CAD build for the part. Positions are in the model's coordinates, mm. A direction names the side the tool comes from. Round coordinates to 2 decimals unless told otherwise and drop trailing zeros. Write each loop counter-clockwise with the first axis right and the second up, starting at its lowest first coordinate (ties: lowest second). Pieces come first, ordered by that corner, then holes. Notation, with made-up numbers: (-26.75, 74.5) -> (18.25, 74.5) arc R32 ccw to (18.25, 109.5) -> close; hole circle Ø8 at (-2, 84.5). An arc over 180 degrees is marked (long way). Put each result on its own line as item: value. Start each with the question number.
1. Saw through at C-C on x = 0.55. State how many separate pieces and enclosed holes the cut face has, and give its area (3 significant figures).
2. 3-axis set-ups, long thin cutter, end or side, ignore diameter. For faces 4 (the cylindrical face through (1.578, 148.765, -37.068)), 5 (the cylindrical face through (1.578, 84.895, -22.369)): which of +Z, -Z, +X, -X, +Y, -Y reach the whole face in a straight line?
3. Flat gauge pins, fed straight in: P1, Ø9.5, axis at y = 0, z = 0, coming from the +X side; P2, Ø1.5, axis at x = 1, y = 88, coming from the -Z side; P3, Ø1.6, axis at x = 2, y = 45.5, coming from the -Z side. Where does each tip first touch, or does it go through?
4. Drill centre lines: line 1 (Z direction, x = 2.55, y = 0); line 2 (Y direction, x = 2.15, z = -94.5); line 3 (Y direction, x = 2.85, z = -65.5). Where is each one in solid material? Low to high. Write a range as from..to.
5. Saw through at A-A on z = 0. List the corners of the cut face in (x, y), and give its area (3 significant figures).
6. Saw through at D-D on y = 83.5. List the corners of the cut face in (x, z).
7. Saw through at B-B on z = -97. List the corners of the cut face in (x, y).
8. Pull direction Z, two halves, no side cores. Call faces 1 (the cylindrical face through (2, 0, 6)), 2 (the flat face through (0, 114, -32)), 3 (the flat face through (1.578, -0.207, -15.487)): pulls with the +Z half, pulls with the -Z half, needs draft (parallel to the pull), parting line crosses it, or undercut.
from build123d import *

# Parameters (mm, degrees)
EXTRUDE1_DEPTH            = 3.2
SKETCH5_R                 = 6
CHASSIS_MOUNT_HOLES_DEPTH = 244.405812041
SKETCH6_R                 = 4
ENGINE_MOUNT_HOLES_DEPTH  = 244.405812041
SKETCH7_R                 = 6.5
SKETCH7_R_2               = 7.5
BOSS_CLEARANCE_DEPTH      = 244.405812041
FILLET1_R                 = 3
FILLET2_R                 = 2
FILLET4_R                 = 4


with BuildPart() as part:
    # Sketch4 → Extrude1 (new body)
    with BuildSketch(Plane(origin=(0, 0, 0), x_dir=(0, 0, -1), z_dir=(1, 0, 0))):
        with BuildLine():
            Line((57.561676807, 155.782132528), (157.015436102, 171.930964589))
            ThreePointArc((157.015436102, 171.930964589), (170.191569786, 165.878071941), (169.567790519, 151.39156416))
            ThreePointArc((169.567790519, 151.39156416), (167.864843482, 149.829218431), (165.697709708, 149.026420829))
            Line((165.697709708, 149.026420829), (86.516546247, 136.169357202))
            ThreePointArc((86.516546247, 136.169357202), (83.134642067, 136.199619503), (79.956239663, 137.355452467))
            ThreePointArc((79.956239663, 137.355452467), (57.745458436, 139.047132616), (42.376364081, 122.923500175))
            ThreePointArc((42.376364081, 122.923500175), (41.240179336, 120.412740542), (39.600266647, 118.197900576))
            ThreePointArc((39.600266647, 118.197900576), (25.651951648, 95.833503084), (20.780663371, 69.92998369))
            Line((20.780663371, 69.92998369), (20.780663371, 30.61290747))
            ThreePointArc((20.780663371, 30.61290747), (26.962955948, 18.753205297), (20.37053182, 7.116486634))
            Line((20.37053182, 7.116486634), (10.815904153, -7.21222708))
            ThreePointArc((10.815904153, -7.21222708), (-4.092243171, -12.339106447), (-12.982184032, 0.680367435))
            Line((-12.982184032, 0.680367435), (-11.728287792, 24.606132992))
            ThreePointArc((-11.728287792, 24.606132992), (-11.013879957, 26.397161442), (-9.356926136, 27.383399496))
            ThreePointArc((-9.356926136, 27.383399496), (4.476016858, 43.584120766), (-7.587711328, 61.142029063))
            ThreePointArc((-7.587711328, 61.142029063), (-9.132498235, 62.296063238), (-9.655779017, 64.1519562))
            ThreePointArc((-9.655779017, 64.1519562), (-0.849075896, 102.602883239), (20.462203873, 135.797177398))
            ThreePointArc((20.462203873, 135.797177398), (37.331902598, 148.908426775), (57.561676807, 155.782132528))
        make_face()
    extrude(amount=EXTRUDE1_DEPTH)

    # Sketch5 → chassis mount holes (cut, through all)
    with BuildSketch(Plane(origin=(0, 0, 0), x_dir=(0, 0, -1), z_dir=(1, 0, 0))):
        Circle(SKETCH5_R)
        with Locations((159.099025767, 159.099025767)):
            Circle(SKETCH5_R)
        with Locations((30.03123526, 126.997538987)):
            Circle(SKETCH5_R)
    extrude(amount=CHASSIS_MOUNT_HOLES_DEPTH, mode=Mode.SUBTRACT)

    # Sketch6 → engine mount holes (cut, through all)
    with BuildSketch(Plane(origin=(0, 0, 0), x_dir=(0, 0, -1), z_dir=(1, 0, 0))):
        with Locations((12.965088215, 18.997538987)):
            Circle(SKETCH6_R)
        with Locations((95.975539476, 147.520941453)):
            Circle(SKETCH6_R)
    extrude(amount=ENGINE_MOUNT_HOLES_DEPTH, mode=Mode.SUBTRACT)

    # Sketch7 → boss clearance (cut, through all)
    with BuildSketch(Plane(origin=(0, 0, 0), x_dir=(0, 0, -1), z_dir=(1, 0, 0))):
        with Locations((139.146474391, 144.715156547)):
            Circle(SKETCH7_R)
        with Locations((33.517273096, 104.769234054)):
            Circle(SKETCH7_R_2)
        Polygon((35.588537275, 119.499655), (44.876445881, 121.763048067), (36.718478427, 114.862903962), align=None)
    extrude(amount=BOSS_CLEARANCE_DEPTH, mode=Mode.SUBTRACT)

    # Fillet1
    fillet1_edges = [part.edges().sort_by_distance(p)[0] for p in [
        (1.6, 30.61290747, -20.780663371),
        (1.6, 7.116486634, -20.37053182),
        (1.6, 143.673361714, -132.730504977),
        (1.6, 145.75695138, -145.562443806),
        (1.6, 100.236921904, -27.541643708),
    ]]
    fillet(fillet1_edges, radius=FILLET1_R)

    # Fillet2
    fillet2_edges = [part.edges().sort_by_distance(p)[0] for p in [
        (1.6, 120.949682485, -41.538773206),
        (1.6, 119.499655, -35.588537275),
    ]]
    fillet(fillet2_edges, radius=FILLET2_R)

    # Fillet4
    fillet4_edges = [part.edges().sort_by_distance(p)[0] for p in [
        (1.6, 114.862903962, -36.718478427),
    ]]
    fillet(fillet4_edges, radius=FILLET4_R)
    fillet4_2_edges = [part.edges().sort_by_distance(p)[0] for p in [
        (1.6, 112.183550135, -34.647723026),
    ]]
    fillet(fillet4_2_edges, radius=FILLET4_R - 0.0001)  # a hair under: the kernel refuses the full size


solid = part.part
Return value:
1. separate pieces: 1
1. enclosed holes: 5
1. area: 6,630 mm^2
2. face 4: +Z, +X, -X, +Y
2. face 5: -Z, +X, -X
3. P1: passes through
3. P2: stops at z = -23.31
3. P3: stops at z = -20.78
4. line 1: z = -15.63..-6, 6..13
4. line 2: y = 137.47..143.8, 151.24..161.78
4. line 3: y = 140.73..157.07
5. outline: (0, -13) -> (3.2, -13) -> (3.2, -6) -> (0, -6) -> close; (0, 6) -> (3.2, 6) -> (3.2, 32.78) -> (0, 32.78) -> close; (0, 56.22) -> (3.2, 56.22) -> (3.2, 104.57) -> (0, 104.57) -> close
5. area: 263 mm^2
6. outline: (0, -22.08) -> (3.2, -22.08) -> (3.2, 6.98) -> (0, 6.98) -> close
7. outline: (0, 137.87) -> (3.2, 137.87) -> (3.2, 143.65) -> (0, 143.65) -> close; (0, 151.39) -> (3.2, 151.39) -> (3.2, 162.19) -> (0, 162.19) -> close
8. face 1: undercut
8. face 2: needs draft
8. face 3: pulls with the -Z half
